Design review of the part built by this model. Coordinates are the model's own, in mm. Face numbers are marked on the shaded views. A direction names the side the tool comes from. Give positions to 0.01 mm unless a question says otherwise; leave off trailing zeros. Loops run counter-clockwise (first coordinate to the right, second up) from the corner with the lowest first, then second, coordinate; pieces in that order, holes last. Notation, with made-up numbers: M -29.75,74.5 L 12.25,74.5 A38 cw 12.25,112.5 Z; hole C 56,-27.75 d2. An arc over 180 degrees is marked long. Use CSV: the item, a comma, the result in double quotes.
from build123d import *

# Parameters (mm, degrees)
F1_DEPTH = 63.5
F2_DEPTH = 25.4
F3_DEPTH = 8.255


with BuildPart() as f1:
    # F0 (on Front) → F1 (new body, symmetric)
    with BuildSketch(Plane.XZ):
        Polygon((22.225, 9.525), (-41.275, 9.525), (-41.275, -9.525), (41.275, -9.525), (41.275, 9.525), align=None)
    extrude(amount=F1_DEPTH, both=True)

    # F0 (on Front) → F2 (join, symmetric)
    with BuildSketch(Plane.XZ):
        with BuildLine():
            Line((22.225, 27.0002), (22.225, 9.525))
            Line((22.225, 9.525), (41.275, 9.525))
            Line((41.275, 9.525), (41.275, 27.0002))
            ThreePointArc((41.275, 27.0002), (45.92468, 38.22552), (57.15, 42.8752))
            Line((57.15, 42.8752), (65.634008, 42.8752))
            Line((65.634008, 42.8752), (65.634008, 61.9252))
            Line((65.634008, 61.9252), (57.15, 61.9252))
            ThreePointArc((57.15, 61.9252), (32.454296, 51.695904), (22.225, 27.0002))
        make_face()
    extrude(amount=F2_DEPTH, both=True)

    # F0 (on Front) → F3 (join, symmetric)
    with BuildSketch(Plane.XZ):
        with BuildLine():
            add(Edge.make_bspline(
                [(-41.275, 9.525), (-31.476464, 46.034317), (42.099748, 66.494018), (65.634008, 61.9252)],
                knots=[0, 0, 0, 0, 119.06014, 119.06014, 119.06014, 119.06014], degree=3))
            Line((-41.275, 9.525), (22.225, 9.525))
            Line((22.225, 9.525), (22.225, 27.0002))
            ThreePointArc((22.225, 27.0002), (32.454296, 51.695904), (57.15, 61.9252))
            Line((57.15, 61.9252), (65.634008, 61.9252))
        make_face()
    extrude(amount=F3_DEPTH, both=True)


solid = f1.part
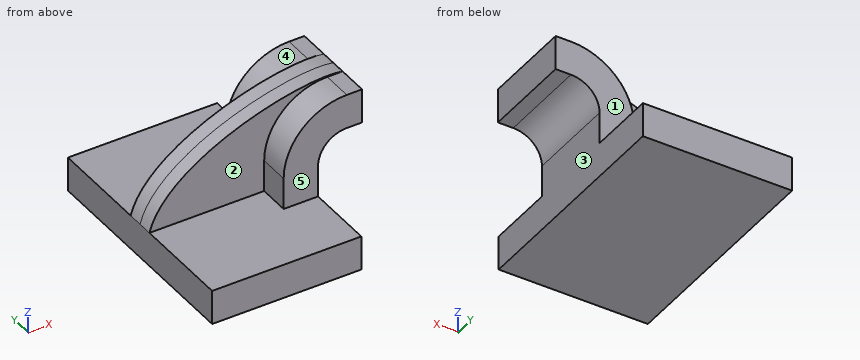
(1) Wall thickness on line 1 along X through (y, z) = (19.5, -0.5) (3 decimals); line 2 along Z through (x, y) = (4, -46) (3 decimals); line 3 along Y through (x, z) = (37.5, 41.5): over which ranges is each line inside the solid? List them lowest first. Write a range as [from, to].
A:
line 1,"[-41.275, 41.275]"
line 2,"[-9.525, 9.525]"
line 3,"[-25.4, 25.4]"
(2) We need section B-B on z = 0. State the section outline as (x, y) points (3 decimals), then the cut area to 3 significant figures.
A:
outline,"M -41.275,-63.5 L 41.275,-63.5 L 41.275,63.5 L -41.275,63.5 Z"
area,"10,500 mm²"
(3) Clearance check with flat-ended pins moving along their axes: P1, Ø4, axis at x = 25, y = 48.5, coming from the +Z side (3 decimals); P2, Ø9.5, axis at x = 60, y = 16.5, coming from the +Z side; P3, Ø10, axis at x = -22.5, z = 19, coming from the +Y side (3 decimals). State where each tip first meets the part, or that it passes through.
A:
P1,"z = 9.525"
P2,"z = 61.93"
P3,"y = 8.255"
(4) Machinability: for the marked faces 1, 2, 3, 4 and 5, which of the approach directions +Z, -Z, +X, -X, +Y, -Y give a long, thin tool a straight path to every point of the face, cutting with its end or side? Answer none if there is none.
A:
face 1,"+Z, +X, -X, +Y"
face 2,"+Z, -X, -Y"
face 3,"-Z, +X, +Y, -Y"
face 4,"+Z, -X, +Y"
face 5,"+Z, +X, -X, -Y"
(5) We need section A-A on y = -18.5. State the section outline as (x, z) points (3 decimals).
A:
outline,"M -41.275,-9.525 L 41.275,-9.525 L 41.275,27 A15.875 cw 57.15,42.875 L 65.634,42.875 L 65.634,61.925 L 57.15,61.925 A34.925 ccw 22.225,27 L 22.225,9.525 L -41.275,9.525 Z"
(6) We need section C-C on y = 53.5. State the section outline as (x, z) points (3 decimals).
A:
outline,"M -41.275,-9.525 L 41.275,-9.525 L 41.275,9.525 L -41.275,9.525 Z"
